```python
from build123d import *

# Parameters (mm, degrees)
F0_R     = 2.947507
F0_R_2   = 2.879107
F0_W     = 31.337534
F0_H     = 28.232014
F1_DEPTH = 12.7
F0_W_2   = 59.569548
F0_H_2   = 9.034242
F2_DEPTH = 25.4
F3_R     = 2.696098
F4_DEPTH = 15
F3_R_2   = 2.610721
F5_DEPTH = 15


with BuildPart() as f1:
    # F0 (on Front) → F1 (new body)
    with BuildSketch(Plane.XZ):
        Polygon((29.784774, 32.043338), (-29.784774, 32.043338), (-29.784774, -41.07758), (-15.668767, -41.07758), (-15.668767, -17.080368), (15.668767, -17.080368), (15.668767, -41.07758), (29.784774, -41.07758), align=None)
        with Locations((-22.72677, -33.454936)):
            Circle(F0_R, mode=Mode.SUBTRACT)
        with Locations((22.72677, -33.454936)):
            Circle(F0_R_2, mode=Mode.SUBTRACT)
        with Locations((0, 11.151646)):
            Rectangle(F0_W, F0_H, mode=Mode.SUBTRACT)
    extrude(amount=F1_DEPTH)

    # F0 (on Front) → F2 (join)
    with BuildSketch(Plane.XZ):
        with Locations((0, 36.560459)):
            Rectangle(F0_W_2, F0_H_2)
    extrude(amount=F2_DEPTH)

    # F3 (on face) → F4 (join)
    with BuildSketch(Plane.XY.offset(41.07758)):
        with Locations((-19.120524, -12.7)):
            Circle(F3_R)
    extrude(amount=F4_DEPTH)

    # F3 (on face) → F5 (join)
    with BuildSketch(Plane.XY.offset(41.07758)):
        with Locations((21.369504, -12.7)):
            Circle(F3_R_2)
    extrude(amount=F5_DEPTH)


solid = f1.part
```
Build history of the part. All positions in model axes, mm. A direction names the side the tool comes from. Round coordinates to 2 decimals unless told otherwise and drop trailing zeros. Write each loop counter-clockwise with the first axis right and the second up, starting at its lowest first coordinate (ties: lowest second). Pieces come first, ordered by that corner, then holes. Notation, with made-up numbers: (33.25, 0) -> (92.25, 0) arc R7 cw to (92.25, 10) -> close; hole circle Ø7 at (-16.5, 0.5). An arc over 180 degrees is marked (long way). Put each result on its own line as item: value.
Item 1: Slice it at B-B, the plane z = 2. Give the cut face in (x, y).
Here are the results:
outline: (-29.78, -12.7) -> (-15.67, -12.7) -> (-15.67, 0) -> (-29.78, 0) -> close; (15.67, -12.7) -> (29.78, -12.7) -> (29.78, 0) -> (15.67, 0) -> close
Item 2: Two-plate mould, pull along X, no slides. Class faces 4 (the face through (23, -6, -41.078)), 5 (the face through (29.785, -7, -1)), 6 (the face through (-20.004, -6.261, -34.584)): pulls with the +X half, pulls with the -X half, needs draft (parallel to the pull), parting line crosses it, or undercut.
Here are the results:
face 4: needs draft
face 5: pulls with the +X half
face 6: undercut
Item 3: Tool access for faces 1 (the face through (0, -19, 32.043)), 2 (the face through (-15.669, -6, -29)), 3 (the face through (0, -6, -2.964)): list every direction of +Z, -Z, +X, -X, +Y, -Y with a clear straight run to the whole face (end or side of a thin tool).
Here are the results:
face 1: -Z, +X, -X, -Y
face 2: -Z, +Y, -Y
face 3: +Y, -Y
Item 4: Wall check: probe 1 along X at (y, z) = (-10, 18); probe 2 along Z at (x, y) = (-6.5, -4); probe 3 along Z at (x, y) = (-0.5, -13). Give the ranges that are in metal, low to high. Write a range as from..to.
Here are the results:
probe 1: x = -29.78..-15.67, 15.67..29.78
probe 2: z = -17.08..-2.96, 25.27..41.08
probe 3: z = 32.04..41.08
Item 5: Slice it at C-C, the plane y = -8.5. Give the cut face in (x, z), plus the area to 3 significant figures.
Here are the results:
outline: (-29.78, -41.08) -> (-15.67, -41.08) -> (-15.67, -17.08) -> (15.67, -17.08) -> (15.67, -41.08) -> (29.78, -41.08) -> (29.78, 41.08) -> (-29.78, 41.08) -> close; hole circle Ø5.9 at (-22.73, -33.45); hole (-15.67, -2.96) -> (15.67, -2.96) -> (15.67, 25.27) -> (-15.67, 25.27) -> close; hole circle Ø5.76 at (22.73, -33.45)
area: 3,200 mm^2
Item 6: Slice it at D-D, the plane x = 17. Give the cut face in (y, z).
Here are the results:
outline: (-25.4, 32.04) -> (-12.7, 32.04) -> (-12.7, -41.08) -> (0, -41.08) -> (0, 41.08) -> (-25.4, 41.08) -> close
Item 7: Flat gauge pins, fed straight in: P1, Ø5, axis at x = 22.73, z = -33.45, coming from the +Y side; P2, Ø3, axis at x = -21, y = -16, coming from the -Z side; P3, Ø6, axis at x = -12.5, z = 27, coming from the -Y side; P4, Ø14, axis at x = 6, y = -4, coming from the +Z side. Where does each tip first touch, or does it go through?
Here are the results:
P1: passes through
P2: stops at z = 32.04
P3: stops at y = -12.7
P4: stops at z = 41.08
Item 8: Slice it at A-A, the plane x = -4. Give the cut face in (y, z).
Here are the results:
outline: (-25.4, 32.04) -> (-12.7, 32.04) -> (-12.7, 25.27) -> (0, 25.27) -> (0, 41.08) -> (-25.4, 41.08) -> close; (-12.7, -17.08) -> (0, -17.08) -> (0, -2.96) -> (-12.7, -2.96) -> close
